from build123d import *

# Parameters (mm, degrees)
BASIS_DEPTH        = 4
MODU_BRACKET_DEPTH = 4
SKETCH3_R          = 5
SKETCH3_W          = 75
SKETCH3_H          = 30
SKETCH3_W_2        = 8
SKETCH3_H_2        = 4
CUT_EXTRUDE2_DEPTH = 5
SKETCH4_W          = 6.1
SKETCH4_H          = 54
CUT_EXTRUDE3_DEPTH = 4
SKETCH5_W          = 4
SKETCH5_H          = 14
CUT_EXTRUDE4_DEPTH = 4
SKETCH6_W          = 10
SKETCH6_H          = 4
CUT_EXTRUDE5_DEPTH = 4
SKETCH9_R          = 1.6
SKETCH9_R_2        = 1.375
CUT_EXTRUDE7_DEPTH = 4
SKETCH10_W         = 30
SKETCH10_H         = 17
CUT_EXTRUDE8_DEPTH = 4
SKETCH11_R         = 1.6
CUT_EXTRUDE9_DEPTH = 4
FILLET1_R          = 3


with BuildPart() as part:
    # Sketch1 → Basis (new body)
    with BuildSketch(Plane(origin=(0, 0, 0), x_dir=(1, 0, 0), z_dir=(0, 1, 0))):
        with BuildLine():
            Line((63.804388564, 77), (-63.804388564, 77))
            ThreePointArc((-63.804388564, 77), (-100, 0), (-63.804388564, -77))
            Line((-63.804388564, -77), (63.804388564, -77))
            ThreePointArc((63.804388564, -77), (90.499831095, -42.541515862), (100, 0))
            ThreePointArc((100, 0), (90.499831095, 42.541515862), (63.804388564, 77))
        make_face()
    extrude(amount=BASIS_DEPTH)

    # Sketch2 → Modu bracket (cut)
    with BuildSketch(Plane(origin=(0, 4, 0), x_dir=(1, 0, 0), z_dir=(0, 1, 0))):
        Polygon((90.817009036, -6.191182133), (94.801787829, -6.539805104), (94.453164858, -10.524583897), (90.468386065, -10.175960926), align=None)
        Polygon((83.047916894, -37.86952889), (86.673148042, -39.560001937), (84.982674995, -43.185233085), (81.357443847, -41.494760038), align=None)
        Polygon((75.166261713, -52.218202052), (78.442869891, -54.512507797), (76.148564145, -57.789115975), (72.871955968, -55.494810229), align=None)
        Polygon((90.468386065, 10.175960926), (94.453164858, 10.524583897), (94.801787829, 6.539805104), (90.817009036, 6.191182133), align=None)
        Polygon((81.357443847, 41.494760038), (84.982674995, 43.185233085), (86.673148042, 39.560001937), (83.047916894, 37.86952889), align=None)
        Polygon((72.871955968, 55.494810229), (76.148564145, 57.789115975), (78.44286989, 54.512507797), (75.166261713, 52.218202052), align=None)
    extrude(amount=-MODU_BRACKET_DEPTH, mode=Mode.SUBTRACT)

    # Sketch3 → Cut-Extrude2 (cut, through all)
    with BuildSketch(Plane(origin=(0, 4, 0), x_dir=(1, 0, 0), z_dir=(0, 1, 0))):
        with Locations((11.304388564, 0)):
            Circle(SKETCH3_R)
        with Locations((11.304388564, -62)):
            Rectangle(SKETCH3_W, SKETCH3_H)
        with Locations((11.304388564, 62)):
            Rectangle(SKETCH3_W, SKETCH3_H)
        with Locations((11.304388564, -37.65)):
            Rectangle(SKETCH3_W_2, SKETCH3_H_2)
        with Locations((11.304388564, 37.65)):
            Rectangle(SKETCH3_W_2, SKETCH3_H_2)
    extrude(amount=-CUT_EXTRUDE2_DEPTH, mode=Mode.SUBTRACT)

    # Sketch4 → Cut-Extrude3 (cut)
    with BuildSketch(Plane(origin=(0, 4, 0), x_dir=(1, 0, 0), z_dir=(0, 1, 0))):
        with BuildLine():
            Line((56.282145861, -18.75), (56.282145861, 18.75))
            ThreePointArc((56.282145861, 18.75), (57.882145861, 20.35), (59.482145861, 18.75))
            Line((59.482145861, 18.75), (59.482145861, -18.75))
            ThreePointArc((59.482145861, -18.75), (57.882145861, -20.35), (56.282145861, -18.75))
        make_face()
        with Locations((78.482145861, 0)):
            Rectangle(SKETCH4_W, SKETCH4_H)
        with Locations((37.282145861, 0)):
            Rectangle(SKETCH4_W, SKETCH4_H)
    extrude(amount=-CUT_EXTRUDE3_DEPTH, mode=Mode.SUBTRACT)

    # Sketch5 → Cut-Extrude4 (cut)
    with BuildSketch(Plane(origin=(0, 4, 0), x_dir=(1, 0, 0), z_dir=(0, 1, 0))):
        with Locations((-1.695611436, -40.64)):
            Rectangle(SKETCH5_W, SKETCH5_H)
        with Locations((-1.695611436, 40.64)):
            Rectangle(SKETCH5_W, SKETCH5_H)
        with Locations((24.304388564, 40.64)):
            Rectangle(SKETCH5_W, SKETCH5_H)
        with Locations((24.304388564, -40.64)):
            Rectangle(SKETCH5_W, SKETCH5_H)
    extrude(amount=-CUT_EXTRUDE4_DEPTH, mode=Mode.SUBTRACT)

    # Sketch6 → Cut-Extrude5 (cut)
    with BuildSketch(Plane(origin=(0, 4, 0), x_dir=(1, 0, 0), z_dir=(0, 1, 0))):
        Polygon((-62.518054096, 57.592655881), (-59.739420614, 60.470015082), (-66.932818617, 67.416598787), (-69.711452099, 64.539239585), align=None)
        Polygon((-59.739420614, -60.470015082), (-62.518054096, -57.592655881), (-69.711452099, -64.539239585), (-66.932818617, -67.416598787), align=None)
        with Locations((58.804388564, -65)):
            Rectangle(SKETCH6_W, SKETCH6_H)
        with Locations((58.804388564, 65)):
            Rectangle(SKETCH6_W, SKETCH6_H)
    extrude(amount=-CUT_EXTRUDE5_DEPTH, mode=Mode.SUBTRACT)

    # Sketch9 → Cut-Extrude7 (cut)
    with BuildSketch(Plane(origin=(0, 4, 0), x_dir=(1, 0, 0), z_dir=(0, 1, 0))):
        with Locations((-54.695611436, -24)):
            Circle(SKETCH9_R)
        with Locations((-54.695611436, 24)):
            Circle(SKETCH9_R)
        with Locations((0.304388564, 24)):
            Circle(SKETCH9_R)
        with Locations((0.304388564, -24)):
            Circle(SKETCH9_R)
        with Locations((-59.695611436, 39)):
            Circle(SKETCH9_R_2)
        with Locations((-59.695611436, -19)):
            Circle(SKETCH9_R_2)
        with Locations((-59.695611436, 19)):
            Circle(SKETCH9_R_2)
        with Locations((-59.695611436, -39)):
            Circle(SKETCH9_R_2)
    extrude(amount=-CUT_EXTRUDE7_DEPTH, mode=Mode.SUBTRACT)

    # Sketch10 → Cut-Extrude8 (cut)
    with BuildSketch(Plane(origin=(0, 4, 0), x_dir=(1, 0, 0), z_dir=(0, 1, 0))):
        with Locations((-29.695611436, 32.5)):
            Rectangle(SKETCH10_W, SKETCH10_H)
        with Locations((-29.695611436, -32.5)):
            Rectangle(SKETCH10_W, SKETCH10_H)
    extrude(amount=-CUT_EXTRUDE8_DEPTH, mode=Mode.SUBTRACT)

    # Sketch11 → Cut-Extrude9 (cut)
    with BuildSketch(Plane(origin=(0, 4, 0), x_dir=(1, 0, 0), z_dir=(0, 1, 0))):
        with Locations((-87, -20)):
            Circle(SKETCH11_R)
        with Locations((-87, 20)):
            Circle(SKETCH11_R)
    extrude(amount=-CUT_EXTRUDE9_DEPTH, mode=Mode.SUBTRACT)

    # Fillet1
    fillet1_edges = [part.edges().sort_by_distance(p)[0] for p in [
        (48.804388564, 2, 77),
        (-26.195611436, 2, 77),
        (-26.195611436, 2, 47),
        (48.804388564, 2, 47),
        (48.804388564, 2, -77),
        (48.804388564, 2, -47),
        (-26.195611436, 2, -47),
        (-26.195611436, 2, -77),
    ]]
    fillet(fillet1_edges, radius=FILLET1_R)


solid = part.part
Verification items for the finished model (mm, model axes). A direction names the side the tool comes from. Give positions to 0.01 mm unless a question says otherwise; leave off trailing zeros. Write each loop counter-clockwise with the first axis right and the second up, starting at its lowest first coordinate (ties: lowest second). Pieces come first, ordered by that corner, then holes. Notation, with made-up numbers: M 17,-38.75 L 37,-38.75 A19 ccw 37,-20.75 Z; hole C 12,67 d4. An arc over 180 degrees is marked long. Put each result on its own line as item: value. Start each with the question number.
1. Go/stop test with flat-tipped pins: pin 1 Ø10 at (x, z) = (-44, -34) entering from +Y; pin 2 Ø1.2 at (x, y) = (-2.5, 3) entering from -Z; pin 3 Ø2 at (x, y) = (78, 3) entering from +Z; pin 4 Ø1.2 at (y, z) = (2, -39) entering from -X. Record where each tip stops, or that it passes through.
2. Scan lines: line 1 along Z through (x, y) = (-30, 3); line 2 along Z through (x, y) = (62, 2.8); line 3 along X through (y, z) = (0.8, -7.5). Record each from-to range of solid material in increasing order. Write a range as [from, to].
3. Section check A-A (y = 3.05). Give the number of separate pieces and of enclosed holes in the cut face, and give its area (3 significant figures).
4. Set-up check for faces 4 (the face through (-2, 2, -33.64)), 5 (the face through (26.304, 2, 40)), 6 (the face through (92.489, 2.028, 10.353)): record each of +Z, -Z, +X, -X, +Y, -Y from which the full face is reachable in a straight line by a thin tool's end or side.
5. Section check B-B (x = 42.5). Record the cut outline in (y, z), and give its area (3 significant figures).
6. Draft check along X on faces 1 (the face through (59.482, 2, 0)), 2 (the face through (-1, 0, -1)), 3 (the face through (-99.992, 1.972, -1.23)). Enter one of: +X half, -X half, draft (parallel to the pull), parting line (faces both ways), or undercut.
Answer list:
1. pin 1: y = 4
1. pin 2: z = -33.64
1. pin 3: z = 63.8
1. pin 4: x = -92.33
2. line 1: [-77, -41], [-24, 24], [41, 77]
2. line 2: [-77, -67], [-63, 63], [67, 77]
2. line 3: [-99.72, 34.23], [40.33, 56.28], [59.48, 75.43], [81.53, 90.7], [94.72, 99.72]
3. separate pieces: 1
3. enclosed holes: 28
3. area: 20,400 mm2
4. face 4: -Z, +Y, -Y
4. face 5: +Z, +Y, -Y
4. face 6: +Y, -Y
5. outline: M 0,-47 L 4,-47 L 4,47 L 0,47 Z
5. area: 376 mm2
6. face 1: undercut
6. face 2: draft
6. face 3: -X half
